Autodesk Inventor part; units mm, degrees
ref_plane "YZ Plane" through (0, 0, 0) normal (1, 0, 0) x (0, 1, 0)
ref_plane "XZ Plane" through (0, 0, 0) normal (0, 1, 0) x (-1, 0, 0)
ref_plane "XY Plane" through (0, 0, 0) normal (0, 0, 1) x (1, 0, 0)
sketch "Sketch1" plane through (0, 0, 0) normal (0, 0, 1) x (1, 0, 0)
  line L0 (-20, 10) -> (20, 10)
  line L1 (20, 10) -> (20, -10)
  line L2 (-20, -10) -> (-20, 10)
  arc A0 (5, -10) -> (-5, -10) centre (0, -10) ccw
  line L3 (20, -10) -> (5, -10)
  line L4 (-5, -10) -> (-20, -10)
  point P0 (0, 0)
  dimension "d0" = 40
  dimension "d1" = 20
  dimension "d2" = 20
  dimension "d3" = 10
  dimension "d4" = 10
  dimension "d5" = 20
  dimension "d6" = 20
  dimension "d7" = 15
extrude "Extrusion1" add sketch "Sketch1" along normal blind 2.6568
sketch "Sketch2" plane through (0, 0, 2.6568) normal (0, 0, 1) x (1, 0, 0)
  line L0 (20, 10) -> (-20, 10)
  line L1 (-20, 10) -> (-20, -10)
  circle A0 centre (-10, 0) radius 2.75
  circle A1 centre (10, 0) radius 2.75
  point P0 (0, 0)
  dimension "d23" = 5.5
  dimension "d24" = 10
  dimension "d25" = 10
  dimension "d28" = 20
extrude "Extrusion2" cut sketch "Sketch2" against normal through all
fillet "Fillet1" radius 2 4 edges at (20, -10, 1.3284) (-20, -10, 1.3284) (-5, -10, 1.3284) (5, -10, 1.3284)
fillet "Fillet2" radius 2 2 edges at (20, 10, 1.3284) (-20, 10, 1.3284)
equation "\"d25\" = d24"
properties part number "30289-01" material "Steel, Mild"
Part model, mm, in its own coordinate system. A direction names the side the tool comes from. Round coordinates to 2 decimals unless told otherwise and drop trailing zeros. Loops run counter-clockwise (first coordinate to the right, second up) from the corner with the lowest first, then second, coordinate; pieces in that order, holes last. Notation, with made-up numbers: (54, 78) -> (104, 78) arc R16 ccw to (104, 88) -> close; hole circle Ø4 at (41, -13). An arc over 180 degrees is marked (long way). Use one line per item in the form item = value. Start each with the question number.
Item 1: Band-saw the part on B-B (z = 0.7). List the corners of the cut face in (x, y).
Item 2: Tool access for faces 1 (the cylindrical face through (-19.43, -9.4, 1.35)), 2 (the cylindrical face through (5.499, -9.593, 1.347)): list every direction of +Z, -Z, +X, -X, +Y, -Y with a clear straight run to the whole face (end or side of a thin tool).
Item 3: Band-saw the part on D-D (x = -9). List the corners of the cut face in (y, z), plus the area to 3 significant figures.
Item 4: Band-saw the part on C-C (x = 10). List the corners of the cut face in (y, z).
Item 5: Drill centre lines: line 1 along Y through (x, z) = (-10, 2.1); line 2 along X through (y, z) = (0.75, 1.05); line 3 along X through (y, z) = (2.5, 2.55). Where is each one in solid material? Low to high.
Item 6: Two-plate mould, pull along X, no slides. Class faces 3 (the cylindrical face through (0, -5, 1)), 4 (the flat face through (-12, -10, 1)), 5 (the cylindrical face through (-7.46, -1.05, 1.35)), 6 (the cylindrical face through (-19.4, 9.43, 1.35)): released by +X, released by -X, zero draft, split by the parting line, or undercut.
Item 7: Band-saw the part on A-A (y = -1). List the corners of the cut face in (x, z).
Item 8: Drop flat-ended pins along their axis: pin 1 Ø5 at (x, y) = (10, 0) entering from -Z; pin 2 Ø5 at (x, y) = (-1, 6) entering from -Z. Give the stop position or say it passes through.
Data:
q1.outline = (-20, -8) arc R2 ccw to (-18, -10) -> (-6.71, -10) arc R2 ccw to (-4.79, -8.57) arc R5 cw to (4.79, -8.57) arc R2 ccw to (6.71, -10) -> (18, -10) arc R2 ccw to (20, -8) -> (20, 8) arc R2 ccw to (18, 10) -> (-18, 10) arc R2 ccw to (-20, 8) -> close; hole circle Ø5.5 at (-10, 0); hole circle Ø5.5 at (10, 0)
q2.face_1 = +Z, -Z, -X, -Y
q2.face_2 = +Z, -Z, -Y
q3.outline = (-10, 0) -> (-2.56, 0) -> (-2.56, 2.66) -> (-10, 2.66) -> close; (2.56, 0) -> (10, 0) -> (10, 2.66) -> (2.56, 2.66) -> close
q3.area = 39.5 mm^2
q4.outline = (-10, 0) -> (-2.75, 0) -> (-2.75, 2.66) -> (-10, 2.66) -> close; (2.75, 0) -> (10, 0) -> (10, 2.66) -> (2.75, 2.66) -> close
q5.line_1 = -10 to -2.75, 2.75 to 10
q5.line_2 = -20 to -12.65, -7.35 to 7.35, 12.65 to 20
q5.line_3 = -20 to -11.15, -8.85 to 8.85, 11.15 to 20
q6.face_3 = undercut
q6.face_4 = zero draft
q6.face_5 = undercut
q6.face_6 = released by -X
q7.outline = (-20, 0) -> (-12.56, 0) -> (-12.56, 2.66) -> (-20, 2.66) -> close; (-7.44, 0) -> (7.44, 0) -> (7.44, 2.66) -> (-7.44, 2.66) -> close; (12.56, 0) -> (20, 0) -> (20, 2.66) -> (12.56, 2.66) -> close
q8.pin_1 = through
q8.pin_2 = 0
